Here's how the part is built. I have some questions about the finished solid (model axes, mm). Face numbers are marked on the shaded views. A direction names the side the tool comes from. Coordinates: 2 decimals unless noted, no trailing zeros. Order: outer loops, then holes, each group sorted by start corner. A loop starts at its lowest first (then second) coordinate and runs counter-clockwise, first axis right, second up.
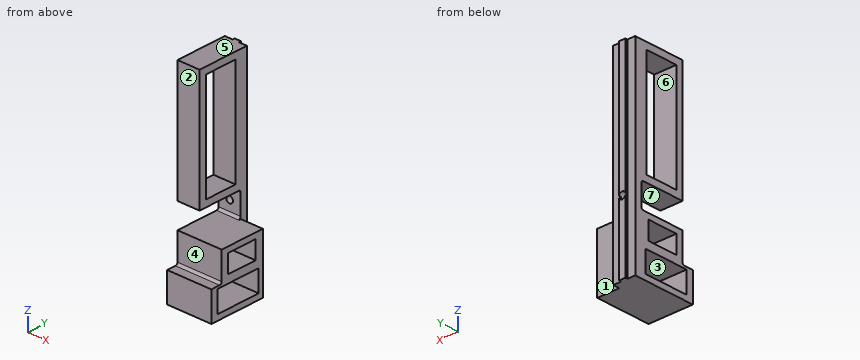
```python
from build123d import *

# Parameters (mm, degrees)
MAKERBEAMFIX_DEPTH            = 45
SKETCH2_R                     = 1.5
MAKERBEAMFIXHOLE_DEPTH        = 5
SKETCH3_W                     = 13
SKETCH3_H                     = 25
SKETCH3_W_2                   = 9.5
SKETCH3_H_2                   = 20
MAKERBEAMTOOLPLATEPLIER_DEPTH = 20
SKETCH4_W                     = 13
SKETCH4_H                     = 20
SKETCH4_W_2                   = 8
SKETCH4_H_2                   = 13.5
MAKERBEAMTOOLCUTPLIER_DEPTH   = 20
SKETCH5_W                     = 53
SKETCH5_H                     = 20
SKETCH5_W_2                   = 47
SKETCH5_H_2                   = 14.5
BIGFACOMPLIER_DEPTH           = 10
FILLET1_R                     = 1


with BuildPart() as part:
    # Sketch1 → MakerBeamFix (new body, symmetric)
    with BuildSketch(Plane.XY):
        Polygon((-5, 0), (5, 0), (5, 3), (1.45, 3), (1.45, 4), (-1.45, 4), (-1.45, 3), (-5, 3), align=None)
    extrude(amount=MAKERBEAMFIX_DEPTH, both=True)

    # Sketch2 → MakerBeamFixHole (cut, through all)
    with BuildSketch(Plane(origin=(0, 0, 0), x_dir=(-1, 0, 0), z_dir=(0, -1, 0))):
        with Locations((0, 13.5)):
            Circle(SKETCH2_R)
    extrude(amount=-MAKERBEAMFIXHOLE_DEPTH, mode=Mode.SUBTRACT)

    # Sketch3 → MakerBeamToolPlatePlier (add)
    with BuildSketch(Plane.ZY.offset(5)):
        with Locations((-38.5, -12.5)):
            Rectangle(SKETCH3_W, SKETCH3_H)
        with Locations((-37.75, -12)):
            Rectangle(SKETCH3_W_2, SKETCH3_H_2, mode=Mode.SUBTRACT)
    extrude(amount=-MAKERBEAMTOOLPLATEPLIER_DEPTH)

    # Sketch4 → MakerBeamToolCutPlier (add)
    with BuildSketch(Plane.ZY.offset(5)):
        with Locations((-25.5, -10)):
            Rectangle(SKETCH4_W, SKETCH4_H)
        with Locations((-25.5, -10.25)):
            Rectangle(SKETCH4_W_2, SKETCH4_H_2, mode=Mode.SUBTRACT)
    extrude(amount=-MAKERBEAMTOOLCUTPLIER_DEPTH)

    # Sketch5 → BigFacomPlier (add)
    with BuildSketch(Plane.ZY.offset(5)):
        with Locations((18.5, -10)):
            Rectangle(SKETCH5_W, SKETCH5_H)
        with Locations((18.5, -9.75)):
            Rectangle(SKETCH5_W_2, SKETCH5_H_2, mode=Mode.SUBTRACT)
    extrude(amount=-BIGFACOMPLIER_DEPTH)

    # Fillet1
    fillet1_edges = [part.edges().sort_by_distance(p)[0] for p in [
        (0, 0, -19),
        (5, -20, -32),
        (0, 0, -8),
    ]]
    fillet(fillet1_edges, radius=FILLET1_R)


solid = part.part
```
Q1. If we section it at D-D on y = -18.5: Write out the boundary of the cut face in (x, z), then the cut area to 3 significant figures.
Q2. I need wall thicknesses on L1, parallel to Z at x = 1.25, y = -18.75; L2, parallel to Z at x = 6, y = -14; L3, parallel to Z at x = 1, y = -9.5. Which ranges of each line are inside material? Lowest first, please.
Q3. We'd pull the mould along Z, two halves only. Please class the marked faces 4, 5, 6 and 7: pulls with the +Z half, pulls with the -Z half, needs draft (parallel to the pull), parting line crosses it, or undercut.
Q4. For the marked faces 1, 2 and 3, which set-ups out of +Z, -Z, +X, -X, +Y, -Y let a thin tool reach every point of the face, with its end or its side?
Q5. If we section it at C-C on x = 0: Give the number of separate pieces and of enclosed holes in the cut face, then the cut area to 3 significant figures.
Q6. Will these pins go through, and if not, where does the flat tip stop? pin 1 (3 mm diameter, centred on x = 6, z = -38.5, fed in from +Y); pin 2 (1.5 mm diameter, centred on y = 1, z = 7.5, fed in from +X); pin 3 (7 mm diameter, centred on x = -2, z = -12.5, fed in from -Y).
Q7. If we section it at A-A on y = -4.5: Write out the boundary of the cut face in (x, z).
Q8. If we section it at B-B on z = -35.5: Write out the boundary of the cut face in (x, y), then the cut area to 3 significant figures.
Reply:
1. outline: (-5, -45) - (15, -45) - (15, -42.5) - (-5, -42.5) - close; (-5, -33) - (15, -33) - (15, -19) - (-5, -19) - close; (-5, -8) - (5, -8) - (5, 45) - (-5, 45) - close
1. area: 860 mm2
2. L1: z = -45 to -42.5, -33 to -19, -8 to 45
2. L2: z = -45 to -42.5, -33 to -29.5, -21.5 to -19
2. L3: z = -45 to -42.5, -33 to -29.5, -21.5 to -19, -8 to -5, 42 to 45
3. face 4: needs draft
3. face 5: pulls with the +Z half
3. face 6: undercut
3. face 7: undercut
4. face 1: +Z, -Z, +X, +Y
4. face 2: +Z, +X, -X, -Y
4. face 3: +X, -X
5. separate pieces: 2
5. enclosed holes: 3
5. area: 1,010 mm2
6. pin 1: stops at y = 3
6. pin 2: stops at x = 5
6. pin 3: stops at y = 0
7. outline: (-5, -45) - (15, -45) - (15, -42.5) - (-5, -42.5) - close; (-5, -33) - (15, -33) - (15, -29.5) - (-5, -29.5) - close; (-5, -21.5) - (15, -21.5) - (15, -19) - (-5, -19) - close; (-5, -8) - (5, -8) - (5, -5) - (-5, -5) - close; (-5, 42) - (5, 42) - (5, 45) - (-5, 45) - close
8. outline: (-5, -25) - (15, -25) - (15, -22) - (-5, -22) - close; (-5, -2) - (15, -2) - (15, 0) - (5, 0) - (5, 3) - (1.45, 3) - (1.45, 4) - (-1.45, 4) - (-1.45, 3) - (-5, 3) - close
8. area: 133 mm2
